from build123d import *

# Parameters (mm, degrees)
F1_DEPTH = 3.175
F0_R     = 1.5875
F2_DEPTH = 1.5875
F3_R     = 0.39624


with BuildPart() as f1:
    # F0 (on Top) → F1 (new body)
    with BuildSketch(Plane.XY):
        with BuildLine():
            ThreePointArc((11.1125, 0), (-4.2525696422, 10.266611305), (-7.8577241059, -7.8577241059))
            ThreePointArc((-7.8577241059, -7.8577241059), (4.2525696422, -10.266611305), (11.1125, 0))
        make_face()
        with BuildLine():
            ThreePointArc((6.35, 0), (2.4300397955, -5.8666350314), (-4.4901280605, -4.4901280605))
            ThreePointArc((-4.4901280605, -4.4901280605), (-2.4300397955, 5.8666350314), (6.35, 0))
        make_face(mode=Mode.SUBTRACT)
    extrude(amount=F1_DEPTH)

    # F0 (on Top) → F2 (join)
    with BuildSketch(Plane.XY):
        with BuildLine():
            ThreePointArc((10.0508463237, -5.8576301025), (11.2306466353, -3.0337960369), (11.6332, 0))
            ThreePointArc((11.6332, 0), (11.2306466353, 3.0337960369), (10.0508463237, 5.8576301025))
            ThreePointArc((10.0508463237, 5.8576301025), (8.2259146069, 8.2259146069), (5.8576301025, 10.0508463237))
            ThreePointArc((5.8576301025, 10.0508463237), (0, 11.6332), (-5.8576301025, 10.0508463237))
            ThreePointArc((-5.8576301025, 10.0508463237), (-8.2259146069, 8.2259146069), (-10.0508463237, 5.8576301025))
            ThreePointArc((-10.0508463237, 5.8576301025), (-11.6332, 0), (-10.0508463237, -5.8576301025))
            ThreePointArc((-10.0508463237, -5.8576301025), (-9.2147810827, -7.1006444664), (-8.2259146069, -8.2259146069))
            ThreePointArc((-8.2259146069, -8.2259146069), (-7.1006444664, -9.2147810827), (-5.8576301025, -10.0508463237))
            ThreePointArc((-5.8576301025, -10.0508463237), (0, -11.6332), (5.8576301025, -10.0508463237))
            ThreePointArc((5.8576301025, -10.0508463237), (8.2259146069, -8.2259146069), (10.0508463237, -5.8576301025))
        make_face()
        with BuildLine():
            ThreePointArc((11.1125, 0), (4.2525696422, -10.266611305), (-7.8577241059, -7.8577241059))
            ThreePointArc((-7.8577241059, -7.8577241059), (-4.2525696422, 10.266611305), (11.1125, 0))
        make_face(mode=Mode.SUBTRACT)
        with BuildLine():
            ThreePointArc((-10.0508463237, 5.8576301025), (-8.2259146069, 8.2259146069), (-5.8576301025, 10.0508463237))
            add(Edge.make_bspline(
                [(-10.31875, 13.890625), (-10.1877713535, 13.556132491), (-9.8378118548, 12.6624079499), (-7.2130077738, 9.6441879633), (-6.2171876005, 9.9429671209), (-5.8576301025, 10.0508463237)],
                knots=[0, 0, 0, 0, 0.2764969064, 0.7387671297, 1, 1, 1, 1], degree=3))
            Line((-10.31875, 13.890625), (-10.31875, 10.31875))
            Line((-10.31875, 10.31875), (-13.890625, 10.31875))
            add(Edge.make_bspline(
                [(-13.890625, 10.31875), (-13.556132491, 10.1877713535), (-12.6624079499, 9.8378118548), (-9.6441879633, 7.2130077738), (-9.9429671209, 6.2171876005), (-10.0508463237, 5.8576301025)],
                knots=[0, 0, 0, 0, 0.2764969064, 0.7387671297, 1, 1, 1, 1], degree=3))
        make_face()
        Polygon((-10.31875, 10.31875), (-10.31875, 13.890625), (-10.31875, 15.08125), (-15.08125, 15.08125), (-15.08125, 10.31875), (-13.890625, 10.31875), align=None)
        with Locations((-12.7, 12.7)):
            Circle(F0_R, mode=Mode.SUBTRACT)
        with BuildLine():
            ThreePointArc((5.8576301025, 10.0508463237), (8.2259146069, 8.2259146069), (10.0508463237, 5.8576301025))
            add(Edge.make_bspline(
                [(13.890625, 10.31875), (13.556132491, 10.1877713535), (12.6624079499, 9.8378118548), (9.6441879633, 7.2130077738), (9.9429671209, 6.2171876005), (10.0508463237, 5.8576301025)],
                knots=[0, 0, 0, 0, 0.2764969064, 0.7387671297, 1, 1, 1, 1], degree=3))
            Line((13.890625, 10.31875), (10.31875, 10.31875))
            Line((10.31875, 10.31875), (10.31875, 13.890625))
            add(Edge.make_bspline(
                [(10.31875, 13.890625), (10.1877713535, 13.556132491), (9.8378118548, 12.6624079499), (7.2130077738, 9.6441879633), (6.2171876005, 9.9429671209), (5.8576301025, 10.0508463237)],
                knots=[0, 0, 0, 0, 0.2764969064, 0.7387671297, 1, 1, 1, 1], degree=3))
        make_face()
        Polygon((10.31875, 10.31875), (13.890625, 10.31875), (15.08125, 10.31875), (15.08125, 15.08125), (10.31875, 15.08125), (10.31875, 13.890625), align=None)
        with Locations((12.7, 12.7)):
            Circle(F0_R, mode=Mode.SUBTRACT)
        with BuildLine():
            add(Edge.make_bspline(
                [(13.890625, -10.31875), (13.556132491, -10.1877713535), (12.6624079499, -9.8378118548), (9.6441879633, -7.2130077738), (9.9429671209, -6.2171876005), (10.0508463237, -5.8576301025)],
                knots=[0, 0, 0, 0, 0.2764969064, 0.7387671297, 1, 1, 1, 1], degree=3))
            ThreePointArc((10.0508463237, -5.8576301025), (8.2259146069, -8.2259146069), (5.8576301025, -10.0508463237))
            add(Edge.make_bspline(
                [(10.31875, -13.890625), (10.1877713535, -13.556132491), (9.8378118548, -12.6624079499), (7.2130077738, -9.6441879633), (6.2171876005, -9.9429671209), (5.8576301025, -10.0508463237)],
                knots=[0, 0, 0, 0, 0.2764969064, 0.7387671297, 1, 1, 1, 1], degree=3))
            Line((10.31875, -13.890625), (10.31875, -10.31875))
            Line((10.31875, -10.31875), (13.890625, -10.31875))
        make_face()
        Polygon((15.08125, -10.31875), (13.890625, -10.31875), (10.31875, -10.31875), (10.31875, -13.890625), (10.31875, -15.08125), (15.08125, -15.08125), align=None)
        with Locations((12.7, -12.7)):
            Circle(F0_R, mode=Mode.SUBTRACT)
        with BuildLine():
            add(Edge.make_bspline(
                [(-10.31875, -13.890625), (-10.1877713535, -13.556132491), (-9.8378118548, -12.6624079499), (-7.2130077738, -9.6441879633), (-6.2171876005, -9.9429671209), (-5.8576301025, -10.0508463237)],
                knots=[0, 0, 0, 0, 0.2764969064, 0.7387671297, 1, 1, 1, 1], degree=3))
            ThreePointArc((-5.8576301025, -10.0508463237), (-7.1006444664, -9.2147810827), (-8.2259146069, -8.2259146069))
            Line((-8.2259146069, -8.2259146069), (-10.31875, -10.31875))
            Line((-10.31875, -10.31875), (-10.31875, -13.890625))
        make_face()
        with BuildLine():
            Line((-10.31875, -10.31875), (-8.2259146069, -8.2259146069))
            ThreePointArc((-8.2259146069, -8.2259146069), (-9.2147810827, -7.1006444664), (-10.0508463237, -5.8576301025))
            add(Edge.make_bspline(
                [(-13.890625, -10.31875), (-13.556132491, -10.1877713535), (-12.6624079499, -9.8378118548), (-9.6441879633, -7.2130077738), (-9.9429671209, -6.2171876005), (-10.0508463237, -5.8576301025)],
                knots=[0, 0, 0, 0, 0.2764969064, 0.7387671297, 1, 1, 1, 1], degree=3))
            Line((-13.890625, -10.31875), (-10.31875, -10.31875))
        make_face()
        Polygon((-10.31875, -15.08125), (-10.31875, -13.890625), (-10.31875, -10.31875), (-13.890625, -10.31875), (-15.08125, -10.31875), (-15.08125, -15.08125), align=None)
        with BuildLine():
            ThreePointArc((-11.1125, -12.7), (-14.1666587579, -13.3075099489), (-11.5774679849, -11.5774679849))
            ThreePointArc((-11.5774679849, -11.5774679849), (-11.2333412421, -12.0924900511), (-11.1125, -12.7))
        make_face(mode=Mode.SUBTRACT)
    extrude(amount=F2_DEPTH)

    # F3
    f3_edges = [f1.edges().sort_by_distance(p)[0] for p in [
        (7.857724, 7.857724, 1.5875),
        (-7.857724, -7.857724, 2.38125),
        (7.857724, 7.857724, 3.175),
    ]]
    fillet(f3_edges, radius=F3_R)


solid = f1.part
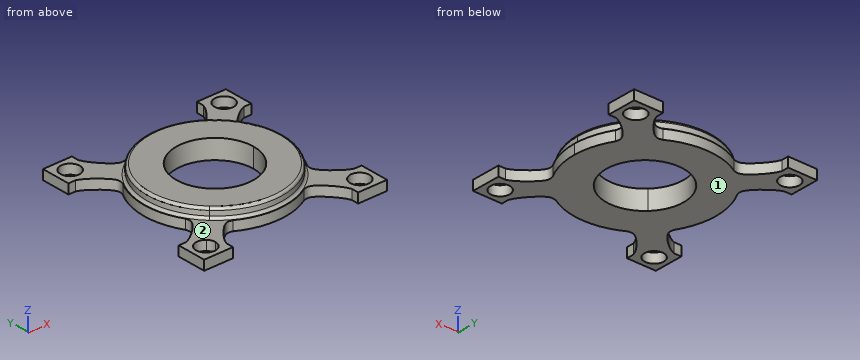
CAD build for the part. Positions are in the model's coordinates, mm. Face numbers are marked on the shaded views. A direction names the side the tool comes from. Coordinates: 2 decimals unless noted, no trailing zeros.
Item 1: 3-axis set-ups, long thin cutter, end or side, ignore diameter. For the marked faces 1 and 2: which of +Z, -Z, +X, -X, +Y, -Y reach the whole face in a straight line?
Check sheet entries:
face 1: -Z, +X, -X, +Y, -Y
face 2: +Z
Item 2: Band-saw the part on A-A on z = 0.35. Give the number of separate pieces and of enclosed holes in the cut face, plus the area to 3 significant figures.
Check sheet entries:
separate pieces: 1
enclosed holes: 5
area: 425 mm2
Item 3: Pin check, flat tips, straight feed: pin 1 Ø5 at (x, y) = (-12.7, 12.7) entering from +Z; pin 2 Ø1 at (y, z) = (3.5, 0.5) entering from +X. Stop position of each tip, or through.
Check sheet entries:
pin 1: stops at z = 1.59
pin 2: stops at x = 11.24
Item 4: Drill centre lines: L1, parallel to X at y = -12.5, z = 0.3; L2, parallel to Y at x = 12.7, z = 0.8; L3, parallel to X at y = -5, z = 2.2. Where is each one in solid material? Low to high.
Check sheet entries:
L1: x = -15.08 to -14.27, -11.13 to -9.56, 9.56 to 11.13, 14.27 to 15.08
L2: y = -15.08 to -14.29, -11.11 to -9.7, 9.7 to 11.11, 14.29 to 15.08
L3: x = -9.92 to -3.91, 3.91 to 9.92
